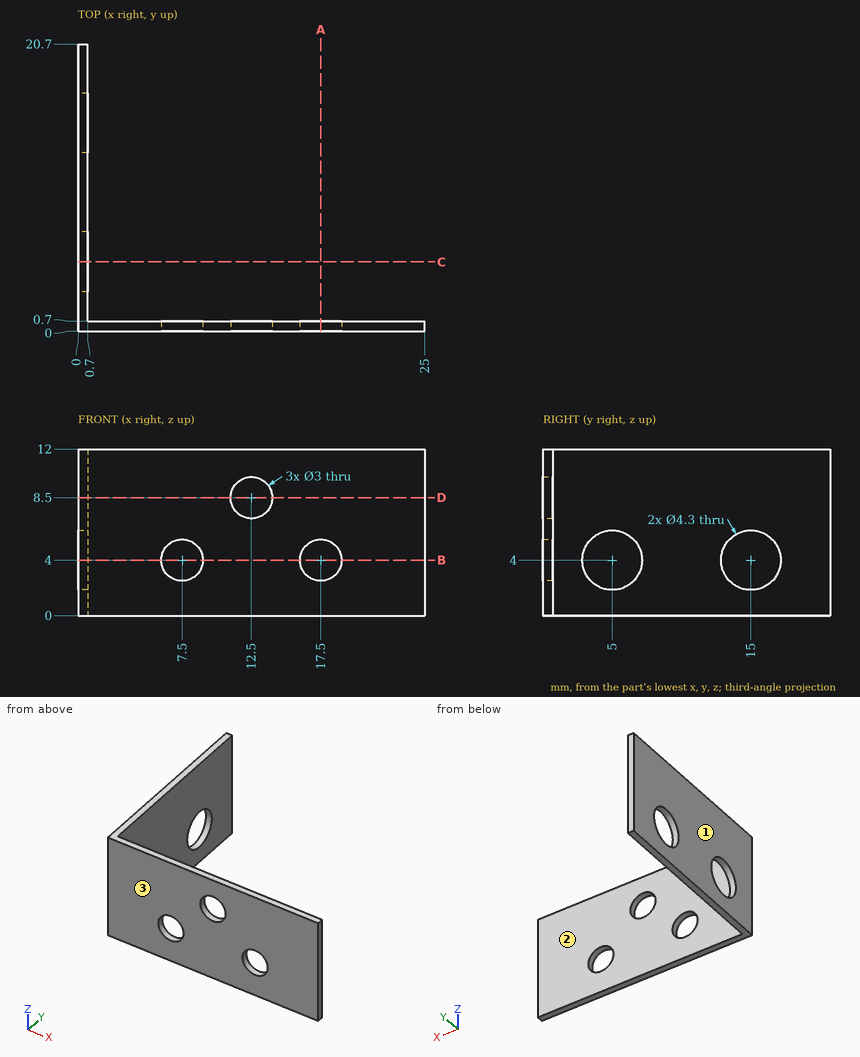
Design review of the part shown in the three views and the two pictorial views. Dimensions are in mm from the part's minimum x, y and z. Round coordinates to 2 decimals unless told otherwise and drop trailing zeros. Order: outer loops, then holes, each group sorted by start corner. A loop starts at its lowest first (then second) coordinate and runs counter-clockwise, first axis right, second up. Notation, with made-up numbers: M 50,-21.75 L 56,-21.75 A24 cw 56,9.25 Z; hole C 59,-18 d6. An arc over 180 degrees is marked long. Put each result on its own line as item: value.
Q1. Insertion check: pin 1 Ø5 at (x, z) = (12.5, 8.5) entering from -Y; pin 2 Ø5 at (y, z) = (10.5, 2.5) entering from +X; pin 3 Ø2.5 at (x, z) = (17.5, 4) entering from -Y. Each pin has a flat end and moves straight along its axis. Give the tip position at first contact, or say it passes through.
Reported:
pin 1: y = 0
pin 2: x = 0.7
pin 3: through
Q2. Consider section C-C (y = 5). State the section outline as (x, z) points, and give its area (3 significant figures).
Reported:
outline: M 0,0 L 0.7,0 L 0.7,1.85 L 0,1.85 Z; M 0,6.15 L 0.7,6.15 L 0.7,12 L 0,12 Z
area: 5.39 mm²
Q3. Consider section A-A (x = 17.5). State the section outline as (y, z) points.
Reported:
outline: M 0,0 L 0.7,0 L 0.7,2.5 L 0,2.5 Z; M 0,5.5 L 0.7,5.5 L 0.7,12 L 0,12 Z
Q4. Draft analysis for pull direction Y (two halves, no side actions). For the marked faces 1, 2 and 3, state which applies: released by +Y, released by -Y, zero draft, split by the parting line, or undercut.
Reported:
face 1: zero draft
face 2: released by +Y
face 3: released by -Y
Q5. Consider section D-D (z = 8.5). State the section outline as (x, y) points.
Reported:
outline: M 0,0 L 11,0 L 11,0.7 L 0.7,0.7 L 0.7,20.7 L 0,20.7 Z; M 14,0 L 25,0 L 25,0.7 L 14,0.7 Z
Q6. Consider section B-B (z = 4). State the section outline as (x, y) points, and give its area (3 significant figures).
Reported:
outline: M 0,0 L 6,0 L 6,0.7 L 0.7,0.7 L 0.7,2.85 L 0,2.85 Z; M 0,7.15 L 0.7,7.15 L 0.7,12.85 L 0,12.85 Z; M 0,17.15 L 0.7,17.15 L 0.7,20.7 L 0,20.7 Z; M 9,0 L 16,0 L 16,0.7 L 9,0.7 Z; M 19,0 L 25,0 L 25,0.7 L 19,0.7 Z
area: 21.3 mm²
Q7. To check wall thickness, follow line 1 (X direction, y = 0.4, z = 4); line 2 (Y direction, x = 0.4, z = 4); line 3 (X direction, y = 8, z = 11.75). State the ranges of each line that lie inside material, in increasing order.
Reported:
line 1: 0 to 6, 9 to 16, 19 to 25
line 2: 0 to 2.85, 7.15 to 12.85, 17.15 to 20.7
line 3: 0 to 0.7
